from build123d import *

# Parameters (mm, degrees)
SKETCH1_R               = 12.7
BOSS_EXTRUDE1_DEPTH     = 25.4
CUT_EXTRUDE1_START      = 25.4
CUT_EXTRUDE1_DEPTH      = 15.748
SKETCH2_W               = 35.052
SKETCH2_H               = 15.748
CUT_EXTRUDE2_DEPTH      = 61.452
CUT_EXTRUDE2_DEPTH_BACK = 1


with BuildPart() as part:
    # Sketch1 → Boss-Extrude1 (new body, symmetric)
    with BuildSketch(Plane.XY):
        Polygon((-33.528, 44.704), (-33.528, 15.748), (45.72, 15.748), (45.72, 44.320833479), (17.78, 60.452), (-17.78, 60.452), align=None)
        with Locations((0, 38.1)):
            Circle(SKETCH1_R, mode=Mode.SUBTRACT)
        Polygon((-33.528, 15.748), (-33.528, 0), (80.772, 0), (80.772, 24.083551843), (45.72, 44.320833479), (45.72, 15.748), align=None)
    extrude(amount=BOSS_EXTRUDE1_DEPTH, both=True)

    # Sketch1<4> → Cut-Extrude1 (cut)
    with BuildSketch(Plane.XY.offset(CUT_EXTRUDE1_START)):
        Polygon((-33.528, 15.748), (-33.528, 0), (80.772, 0), (80.772, 24.083551843), (45.72, 44.320833479), (45.72, 15.748), align=None)
    extrude(amount=-CUT_EXTRUDE1_DEPTH, mode=Mode.SUBTRACT)

    # Sketch2 → Cut-Extrude2 (cut, two sides)
    with BuildSketch(Plane(origin=(0, 0, 0), x_dir=(1, 0, 0), z_dir=(0, 1, 0))) as cut_extrude2_sk:
        with Locations((47.498, 17.526)):
            Rectangle(SKETCH2_W, SKETCH2_H)
    extrude(amount=CUT_EXTRUDE2_DEPTH, mode=Mode.SUBTRACT)
    extrude(cut_extrude2_sk.sketch, amount=-CUT_EXTRUDE2_DEPTH_BACK, mode=Mode.SUBTRACT)


solid = part.part
Design review of the part built by this model. Coordinates are the model's own, in mm. A direction names the side the tool comes from. Round coordinates to 2 decimals unless told otherwise and drop trailing zeros. Order: outer loops, then holes, each group sorted by start corner. A loop starts at its lowest first (then second) coordinate and runs counter-clockwise, first axis right, second up.
1) Consider section C-C (z = 11.5). State the section outline as (x, y) points, plus the area to 3 significant figures.
The answers:
outline: (-33.53, 15.75) - (45.72, 15.75) - (45.72, 44.32) - (17.78, 60.45) - (-17.78, 60.45) - (-33.53, 44.7) - close; hole circle Ø25.4 at (0, 38.1)
area: 2,690 mm2
2) Consider section B-B (z = -19.5). State the section outline as (x, y) points, plus the area to 3 significant figures.
The answers:
outline: (-33.53, 0) - (29.97, 0) - (29.97, 53.41) - (17.78, 60.45) - (-17.78, 60.45) - (-33.53, 44.7) - close; (65.02, 0) - (80.77, 0) - (80.77, 24.08) - (65.02, 33.18) - close; hole circle Ø25.4 at (0, 38.1)
area: 3,620 mm2
3) Machinability: for faces 4 (the flat face through (7, 15.748, 18)), 5 (the flat face through (47, 20, -9.652)), 6 (the flat face through (73, 13, -25.4)), which of the approach directions +Z, -Z, +X, -X, +Y, -Y give a long, thin tool a straight path to every point of the face, cutting with its end or side? Answer none if there is none.
The answers:
face 4: +Z, +X, -X, -Y
face 5: -Z, +Y, -Y
face 6: -Z, +X, -X, +Y, -Y
4) For L1, parallel to X at y = 38, z = -11; L2, parallel to Y at x = 0, z = 7; L3, parallel to Y at x = 0, z = 13, list the stretches that pass through material, from the lowest coordinate up.
The answers:
L1: x = -33.53 to -12.7, 12.7 to 29.97
L2: y = 0 to 25.4, 50.8 to 60.45
L3: y = 15.75 to 25.4, 50.8 to 60.45
5) Consider section A-A (x = 0). State the section outline as (y, z) points, plus the area to 3 significant figures.
The answers:
outline: (0, -25.4) - (25.4, -25.4) - (25.4, 25.4) - (15.75, 25.4) - (15.75, 9.65) - (0, 9.65) - close; (50.8, -25.4) - (60.45, -25.4) - (60.45, 25.4) - (50.8, 25.4) - close
area: 1,530 mm2
6) Clearance check with flat-ended pins moving along their axes: pin 1 Ø8 at (x, z) = (24.5, 20) entering from -Y; pin 2 Ø12.5 at (y, z) = (27, 18.5) entering from +X; pin 3 Ø8 at (y, z) = (28.5, -14.5) entering from +X. State where each tip first meets the part, or that it passes through.
The answers:
pin 1: stops at y = 15.75
pin 2: stops at x = 45.72
pin 3: stops at x = 80.05
7) Consider section D-D (y = 38.1). State the section outline as (x, z) points, plus the area to 3 significant figures.
The answers:
outline: (-33.53, -25.4) - (-12.7, -25.4) - (-12.7, 25.4) - (-33.53, 25.4) - close; (12.7, -25.4) - (29.97, -25.4) - (29.97, -9.65) - (56.49, -9.65) - (56.49, 9.65) - (45.72, 9.65) - (45.72, 25.4) - (12.7, 25.4) - close
area: 2,700 mm2
8) Draft analysis for pull direction X (two halves, no side actions). For faces 1 (the flat face through (36, 13, 9.652)), 2 (the flat face through (45.72, 30, 18)), 3 (the cylindrical face through (6.827, 48.809, -0.356)), state which applies: released by +X, released by -X, zero draft, split by the parting line, or undercut.
The answers:
face 1: zero draft
face 2: released by +X
face 3: undercut
